```python
from build123d import *

# Parameters (mm, degrees)
F0_R     = 15
F1_DEPTH = 160
F3_DEPTH = 40


# Not quite as in the source:
# - a feature names something its author has since deleted; it is built from what else it names


with BuildPart() as f1:
    # F0 (on Top) → F1 (new body)
    with BuildSketch(Plane.XY):
        Circle(F0_R)
    extrude(amount=F1_DEPTH)

    # F2 (on face) → F3 (cut)
    with BuildSketch(Plane.XY.offset(160)):
        with BuildLine():
            ThreePointArc((-3.25, 9.1923881554), (-5.6291651246, -7.960841664), (9.75, 0))
            ThreePointArc((9.75, 0), (7.960841664, 5.6291651246), (3.25, 9.1923881554))
            Line((3.25, 9.1923881554), (3.25, 6.55))
            Line((3.25, 6.55), (-3.25, 6.55))
            Line((-3.25, 6.55), (-3.25, 9.1923881554))
        make_face()
        with BuildLine():
            Line((3.25, 6.55), (3.25, 9.1923881554))
            ThreePointArc((3.25, 9.1923881554), (0, 9.75), (-3.25, 9.1923881554))
            Line((-3.25, 9.1923881554), (-3.25, 6.55))
            Line((-3.25, 6.55), (3.25, 6.55))
        make_face()
        with BuildLine():
            ThreePointArc((-3.25, 9.1923881554), (0, 9.75), (3.25, 9.1923881554))
            Line((3.25, 9.1923881554), (3.25, 12.95))
            Line((3.25, 12.95), (-3.25, 12.95))
            Line((-3.25, 12.95), (-3.25, 9.1923881554))
        make_face()
    extrude(amount=-F3_DEPTH, mode=Mode.SUBTRACT)


solid = f1.part
```
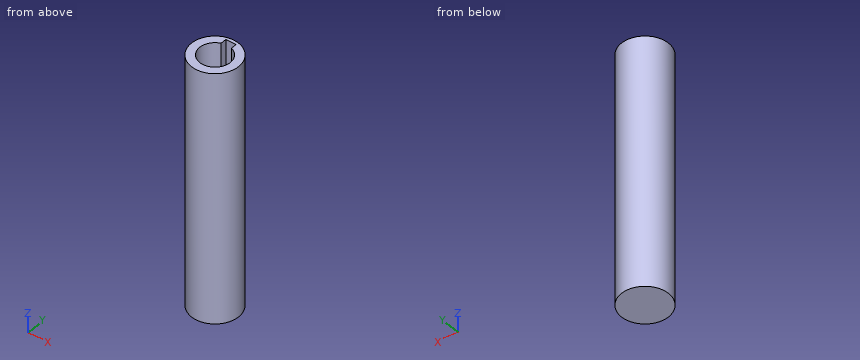
The model under review builds one solid part; all positions refer to its coordinate system, in mm. Coordinates: 2 decimals unless noted, no trailing zeros. Write each loop counter-clockwise with the first axis right and the second up, starting at its lowest first coordinate (ties: lowest second). Pieces come first, ordered by that corner, then holes. Notation, with made-up numbers: (-16.5, 24) - (-10.5, 24) arc R11 cw to (-10.5, 32) - close; hole circle Ø4 at (48.5, 35). An arc over 180 degrees is marked (long way). Answer in a Markdown table with one row per item. Add a question column.
Q1. Clearance check with flat-ended pins moving along their axes: pin 1 (8 mm diameter, centred on x = 1.5, y = -3, fed in from +Z); pin 2 (4 mm diameter, centred on y = 12, z = 144, fed in from +X); pin 3 (4 mm diameter, centred on x = 6.5, z = 54.5, fed in from -Y). State where each tip first meets the part, or that it passes through.
Q2. Consider section B-B on y = 7.5. Give the boundary of the cut face in (x, z).
Q3. Consider section D-D on x = 11.5. Give the boundary of the cut face in (y, z), then the cut area to 3 significant figures.
Q4. Consider section A-A on x = 0. Give the boundary of the cut face in (y, z).
Q5. Consider section C-C on z = 54.5. Give the boundary of the cut face in (x, y), then the cut area to 3 significant figures.
Q6. To check wall thickness, follow line 1 along Y through (x, z) = (0, 141.5); line 2 along Z through (x, y) = (-3.5, -2.5); line 3 along X through (y, z) = (9.5, 147.5). State the ranges of each line that lie inside material, in increasing order. Write a range as from..to.
Answers below:
| question | item | result |
|---|---|---|
| 1 | pin 1 | z = 120 |
| 1 | pin 2 | x = 11.18 |
| 1 | pin 3 | y = -14.31 |
| 2 | outline | (-12.99, 0) - (12.99, 0) - (12.99, 160) - (6.23, 160) - (6.23, 120) - (-6.23, 120) - (-6.23, 160) - (-12.99, 160) - close |
| 3 | outline | (-9.63, 0) - (9.63, 0) - (9.63, 160) - (-9.63, 160) - close |
| 3 | area | 3,080 mm² |
| 4 | outline | (-15, 0) - (15, 0) - (15, 160) - (12.95, 160) - (12.95, 120) - (-9.75, 120) - (-9.75, 160) - (-15, 160) - close |
| 5 | outline | circle Ø30 at (0, 0) |
| 5 | area | 707 mm² |
| 6 | line 1 | -15..-9.75, 12.95..15 |
| 6 | line 2 | 0..120 |
| 6 | line 3 | -11.61..-3.25, 3.25..11.61 |
